Here's how the part is built. I have some questions about the finished solid (model axes, mm). A direction names the side the tool comes from. Give positions to 0.01 mm unless a question says otherwise; leave off trailing zeros. Write each loop counter-clockwise with the first axis right and the second up, starting at its lowest first coordinate (ties: lowest second). Pieces come first, ordered by that corner, then holes. Notation, with made-up numbers: (-17, 35) -> (-5, 35) arc R21 ccw to (-5, 47) -> close; hole circle Ø2 at (33.5, 13.25). An arc over 180 degrees is marked (long way). Return JSON: item names as keys, results as strings.
from build123d import *

# Parameters (mm, degrees)
SKETCH3_R           = 4
BOSS_EXTRUDE1_DEPTH = 15
BOSS_EXTRUDE2_DEPTH = 60
SKETCH6_R           = 3.4
CUT_EXTRUDE1_DEPTH  = 107.024394791
SKETCH7_R           = 4
CUT_EXTRUDE2_DEPTH  = 107.024394862
CUT_EXTRUDE3_START  = -5
SKETCH10_R          = 7
SKETCH10_R_2        = 3.4
CUT_EXTRUDE3_DEPTH  = 102.024394862
BOSS_EXTRUDE3_DEPTH = 15
FILLET1_R           = 1


with BuildPart() as part:
    # Sketch3 → Boss-Extrude1 (new body)
    with BuildSketch(Plane(origin=(0, 0, 0), x_dir=(1, 0, 0), z_dir=(0, 1, 0))):
        with BuildLine():
            ThreePointArc((-50.387748924, -18.119611268), (-46.048367083, 0), (-50.387748924, 18.119611268))
            ThreePointArc((-50.387748924, 18.119611268), (-45.961940777, 45.961940777), (-18.119611268, 50.387748924))
            ThreePointArc((-18.119611268, 50.387748924), (0, 46.048367083), (18.119611268, 50.387748924))
            ThreePointArc((18.119611268, 50.387748924), (45.961940777, 45.961940777), (50.387748924, 18.119611268))
            ThreePointArc((50.387748924, 18.119611268), (46.048367083, 0), (50.387748924, -18.119611268))
            ThreePointArc((50.387748924, -18.119611268), (45.961940777, -45.961940777), (18.119611268, -50.387748924))
            ThreePointArc((18.119611268, -50.387748924), (0, -46.048367083), (-18.119611268, -50.387748924))
            ThreePointArc((-18.119611268, -50.387748924), (-45.961940777, -45.961940777), (-50.387748924, -18.119611268))
        make_face()
        with Locations(Location((28.991378029, 28.991378029, 0), (0, 0, 270))):
            Circle(SKETCH3_R, mode=Mode.SUBTRACT)
        with Locations(Location((28.991378029, -28.991378029, 0), (0, 0, 270))):
            Circle(SKETCH3_R, mode=Mode.SUBTRACT)
        with Locations(Location((-28.991378029, -28.991378029, 0), (0, 0, 270))):
            Circle(SKETCH3_R, mode=Mode.SUBTRACT)
        with Locations(Location((-28.991378029, 28.991378029, 0), (0, 0, 270))):
            Circle(SKETCH3_R, mode=Mode.SUBTRACT)
        with BuildLine():
            Line((-4, 18.7), (-4, 14.456832295))
            ThreePointArc((-4, 14.456832295), (0, -15), (4, 14.456832295))
            Line((4, 14.456832295), (4, 18.7))
            Line((4, 18.7), (-4, 18.7))
        make_face(mode=Mode.SUBTRACT)
    extrude(amount=BOSS_EXTRUDE1_DEPTH)

    # Sketch4 → Boss-Extrude2 (add)
    with BuildSketch(Plane(origin=(0, 15, 0), x_dir=(1, 0, 0), z_dir=(0, 1, 0))):
        with BuildLine():
            Line((-4, 14.456832295), (-4, 18.7))
            Line((-4, 18.7), (4, 18.7))
            Line((4, 18.7), (4, 14.456832295))
            ThreePointArc((4, 14.456832295), (14.945994408, -1.271711896), (1.5, -14.924811557))
            Line((1.5, -14.924811557), (1.5, -29.962476533))
            ThreePointArc((1.5, -29.962476533), (21.737065119, -20.676073128), (30, 0))
            ThreePointArc((30, 0), (-20.676073128, 21.737065119), (-1.5, -29.962476533))
            Line((-1.5, -29.962476533), (-1.5, -14.924811557))
            ThreePointArc((-1.5, -14.924811557), (-14.945994408, -1.271711896), (-4, 14.456832295))
        make_face()
    extrude(amount=BOSS_EXTRUDE2_DEPTH)

    # Sketch6 → Cut-Extrude1 (cut, through all)
    with BuildSketch(Plane(origin=(0, 0, 0), x_dir=(0, 0, -1), z_dir=(1, 0, 0))):
        with Locations(Location((-22.443644045, 65, 0), (0, 0, 180))):
            Circle(SKETCH6_R)
        with Locations(Location((-22.443644045, 45, 0), (0, 0, 180))):
            Circle(SKETCH6_R)
    extrude(amount=CUT_EXTRUDE1_DEPTH, mode=Mode.SUBTRACT)

    # Sketch7 → Cut-Extrude2 (cut, through all)
    with BuildSketch(Plane(origin=(0, 0, 0), x_dir=(0, 0, -1), z_dir=(1, 0, 0))):
        with Locations((-22.443644045, 65)):
            Circle(SKETCH7_R)
        with Locations((-22.443644045, 45)):
            Circle(SKETCH7_R)
    extrude(amount=-CUT_EXTRUDE2_DEPTH, mode=Mode.SUBTRACT)

    # Sketch10 → Cut-Extrude3 (cut, through all)
    # profile 1 of 2: a face of its own
    with BuildSketch(Plane(origin=(0, 0, 0), x_dir=(0, 0, -1), z_dir=(1, 0, 0)).offset(CUT_EXTRUDE3_START)):
        with Locations((-22.443644045, 65)):
            Circle(SKETCH10_R)
        with Locations(Location((-22.443644045, 65, 0), (0, 0, 180))):
            Circle(SKETCH10_R_2, mode=Mode.SUBTRACT)
    # profile 2 of 2: a face of its own
    with BuildSketch(Plane(origin=(0, 0, 0), x_dir=(0, 0, -1), z_dir=(1, 0, 0)).offset(CUT_EXTRUDE3_START)):
        with Locations((-22.443644045, 45)):
            Circle(SKETCH10_R)
        with Locations(Location((-22.443644045, 45, 0), (0, 0, 180))):
            Circle(SKETCH10_R_2, mode=Mode.SUBTRACT)
    extrude(amount=-CUT_EXTRUDE3_DEPTH, mode=Mode.SUBTRACT)

    # Sketch11 → Boss-Extrude3 (add)
    with BuildSketch(Plane(origin=(0, 0, 0), x_dir=(1, 0, 0), z_dir=(0, 1, 0))):
        with BuildLine():
            ThreePointArc((-50.387748924, 18.119611268), (-52.693787753, 32.759105894), (-45.961940644, 45.96194091))
            ThreePointArc((-45.961940644, 45.96194091), (-65, 1.62e-07), (-45.961940873, -45.961940681))
            ThreePointArc((-45.961940873, -45.961940681), (-52.693787778, -32.759105733), (-50.387748924, -18.119611268))
            ThreePointArc((-50.387748924, -18.119611268), (-46.048367083, 0), (-50.387748924, 18.119611268))
        make_face()
        with BuildLine():
            ThreePointArc((18.119611268, 50.387748924), (32.759105845, 52.693787761), (45.961940841, 45.961940713))
            ThreePointArc((45.961940841, 45.961940713), (1.4e-07, 65), (-45.961940644, 45.96194091))
            ThreePointArc((-45.961940644, 45.96194091), (-32.759105708, 52.693787782), (-18.119611268, 50.387748924))
            ThreePointArc((-18.119611268, 50.387748924), (0, 46.048367083), (18.119611268, 50.387748924))
        make_face()
        with BuildLine():
            ThreePointArc((-45.961940873, -45.961940681), (-8.4e-08, -65), (45.961940754, -45.9619408))
            ThreePointArc((45.961940754, -45.9619408), (32.759105785, -52.69378777), (18.119611268, -50.387748924))
            ThreePointArc((18.119611268, -50.387748924), (0, -46.048367083), (-18.119611268, -50.387748924))
            ThreePointArc((-18.119611268, -50.387748924), (-32.759105868, -52.693787757), (-45.961940873, -45.961940681))
        make_face()
        with BuildLine():
            ThreePointArc((45.961940754, -45.9619408), (60.052169607, -24.874423119), (65, 0))
            ThreePointArc((65, 0), (60.052169631, 24.874423062), (45.961940841, 45.961940713))
            ThreePointArc((45.961940841, 45.961940713), (52.693787775, 32.759105756), (50.387748924, 18.119611268))
            ThreePointArc((50.387748924, 18.119611268), (46.048367083, 0), (50.387748924, -18.119611268))
            ThreePointArc((50.387748924, -18.119611268), (52.693787765, -32.759105817), (45.961940754, -45.9619408))
        make_face()
    extrude(amount=BOSS_EXTRUDE3_DEPTH)

    # Fillet1
    fillet1_edges = [part.edges().sort_by_distance(p)[0] for p in [
        (0, 15, -30),
    ]]
    fillet(fillet1_edges, radius=FILLET1_R)


solid = part.part
1. Suppose I cut it at B-B, the plane y = 45. List the corners of the cut face in (x, z) for me.
Taken from the geometry:
{"outline": "(-25.72, 15.44) arc R30 ccw (long way) to (23.18, 19.04) -> (1.5, 19.04) -> (1.5, 14.92) arc R15 cw to (4, -14.46) -> (4, -18.7) -> (-4, -18.7) -> (-4, -14.46) arc R15 cw to (-1.5, 14.92) -> (-1.5, 18.44) -> (-5, 18.44) -> (-5, 15.44) -> close; (-5.75, 29.44) -> (-5, 29.44) -> (-5, 26.44) -> (-1.5, 26.44) -> (-1.5, 29.96) arc R30 ccw to start; (1.5, 25.84) -> (15.24, 25.84) arc R30 ccw to (1.5, 29.96) -> close"}
2. Suppose I cut it at C-C, the plane x = 8.5. Count the separate pieces of the cut face and the enclosed holes in it, and give its area (3 significant figures).
Taken from the geometry:
{"separate pieces": "2", "enclosed holes": "2", "area": "3,460 mm²"}
3. If we mould it in two halves opening along Y, with no side actions, what happens to faces 1 (the face through (9.783, 44.851, 19.047)), 2 (the face through (-1, 15, 28)), 3 (the face through (-5, 62, 19)), 4 (the face through (-30.523, 7.395, -25.296))? For each: released by +Y, released by -Y, zero draft, split by the parting line, or undercut.
Taken from the geometry:
{"face 1": "undercut", "face 2": "released by +Y", "face 3": "undercut", "face 4": "zero draft"}
4. Suppose I cut it at A-A, the plane y = 36. List the corners of the cut face in (x, z) for me.
Taken from the geometry:
{"outline": "(-4, -18.7) -> (-4, -14.46) arc R15 cw to (-1.5, 14.92) -> (-1.5, 29.96) arc R30 ccw (long way) to (1.5, 29.96) -> (1.5, 14.92) arc R15 cw to (4, -14.46) -> (4, -18.7) -> close"}
5. For pin 1 Ø7 at (y, z) = (64, 22) entering from -X; pin 2 Ø7 at (x, z) = (-28.99, 28.99) entering from -Y; pin 3 Ø1 at (x, y) = (2.5, 45) entering from +Z; pin 4 Ø5 at (y, z) = (35, 21.5) entering from +X, each with a flat end and sliding along its axis, tell me the tip position at first contact or that it passes through.
Taken from the geometry:
{"pin 1": "stops at x = -5", "pin 2": "passes through", "pin 3": "stops at z = 29.93", "pin 4": "stops at x = 23.22"}
6. Suppose I cut it at D-D, the plane x = -43. List the corners of the cut face in (y, z) for me.
Taken from the geometry:
{"outline": "(0, -48.74) -> (15, -48.74) -> (15, 48.74) -> (0, 48.74) -> close"}
7. If I drill on line 1 (Z direction, x = 0, y = 11); line 2 (X direction, y = 13.5, z = 26); line 3 (Y direction, x = -34, z = 20), over which ranges is the centre line in solid material (lowest first)? Write a range as [from, to].
Taken from the geometry:
{"line 1": "z = [-65, -18.7], [15, 65]", "line 2": "x = [-59.57, -31.65], [-26.34, 26.34], [31.65, 59.57]", "line 3": "y = [0, 15]"}
8. Which directions (+Z, -Z, +X, -X, +Y, -Y) give clear straight access to the entire face, cutting with the end or side of a thin tool? Please do faces 5 (the face through (-5, 42, 19)), 6 (the face through (-1.5, 45, 27)), 7 (the face through (4, 37, -17)).
Taken from the geometry:
{"face 5": "-X", "face 6": "+Z, +Y", "face 7": "+Y, -Y"}
